Model file for the job. Use its own axes, mm. A direction names the side the tool comes from. Round coordinates to 2 decimals unless told otherwise and drop trailing zeros. Order: outer loops, then holes, each group sorted by start corner. A loop starts at its lowest first (then second) coordinate and runs counter-clockwise, first axis right, second up. Notation, with made-up numbers: (-2.5, -26) - (39.5, -26) arc R22 cw to (39.5, 5) - close; hole circle Ø6 at (51, -26). An arc over 180 degrees is marked (long way). Write item = value, one per line.
```python
from build123d import *

# Parameters (mm, degrees)
F0_W      = 19
F0_H      = 19
F1_DEPTH  = 9.5
F3_DEPTH  = 19.001
F5_DEPTH  = 3
F6_R      = 2
F8_DEPTH  = 12.501
F9_R      = 2
F11_DEPTH = 9.5
F12_R     = 2.99999
F13_R     = 2


# Not quite as in the source:
# - a fillet or chamfer is up to 0.001 mm smaller than in the source, because OpenCascade refuses the exact size


with BuildPart() as f1:
    # F0 (on Front) → F1 (new body, symmetric)
    with BuildSketch(Plane.XZ):
        with Locations((9.5, 9.5)):
            Rectangle(F0_W, F0_H)
    extrude(amount=F1_DEPTH, both=True)

    # F2 (on face) → F3 (cut, through all)
    with BuildSketch(Plane.XZ.offset(9.5)):
        with BuildLine():
            ThreePointArc((6, 19), (9.8076118446, 9.8076118446), (19, 6))
            Line((19, 6), (19, 19))
            Line((19, 19), (6, 19))
        make_face()
    extrude(amount=-F3_DEPTH, mode=Mode.SUBTRACT)

    # F4 (on Front) → F5 (join, symmetric)
    with BuildSketch(Plane.XZ):
        Polygon((0, 18), (0, 0), (18, 0), (18, 11.5), (24.5, 11.5), (24.5, 24.5), (11.5, 24.5), (11.5, 18), align=None)
    extrude(amount=F5_DEPTH, both=True)

    # F6
    f6_edges = [f1.edges().sort_by_distance(p)[0] for p in [
        (0, 0, 0),
    ]]
    fillet(f6_edges, radius=F6_R)

    # F7 (on face) → F8 (cut, through all)
    with BuildSketch(Plane.XZ.offset(3)):
        Polygon((17.5, 24.5), (24.5, 17.5), (24.5, 24.5), align=None)
    extrude(amount=-F8_DEPTH, mode=Mode.SUBTRACT)

    # F9
    f9_edges = [f1.edges().sort_by_distance(p)[0] for p in [
        (0, -9.5, 10.5),
        (0, 9.5, 10.5),
        (0, 0, 19),
        (3, 9.5, 19),
        (3, -9.5, 19),
        (19, 9.5, 3),
        (19, 0, 0),
        (19, -9.5, 3),
    ]]
    fillet(f9_edges, radius=F9_R)

    # F10 (on Front) → F11 (cut, symmetric)
    with BuildSketch(Plane.XZ):
        Polygon((0, 25), (0, 0), (25, 25), align=None)
    extrude(amount=F11_DEPTH, both=True, mode=Mode.SUBTRACT)

    # F12 (radius 3 in the source; OpenCascade refuses exactly that, so slightly less here)
    f12_edges = [f1.edges().sort_by_distance(p)[0] for p in [
        (22.75, -3, 19.25),
        (24.5, -3, 14.5),
        (24.5, 3, 14.5),
        (22.75, 3, 19.25),
    ]]
    fillet(f12_edges, radius=F12_R)

    # F13
    f13_edges = [f1.edges().sort_by_distance(p)[0] for p in [
        (23.579023, 2.162797, 17.118519),
    ]]
    fillet(f13_edges, radius=F13_R)


solid = f1.part
```
1) Cut at A-A (x = 6.5). Write the cut outline in (y, z).
Conclusion:
outline = (-9.5, 2) arc R2 ccw to (-7.5, 0) - (7.5, 0) arc R2 ccw to (9.5, 2) - (9.5, 6.5) - (-9.5, 6.5) - close
2) Cut at D-D (z = 7.5). Write the cut outline in (x, y), and give its area (3 significant figures).
Conclusion:
outline = (7.5, -9.5) - (12.94, -9.5) - (12.94, -3) - (18, -3) - (18, 3) - (12.94, 3) - (12.94, 9.5) - (7.5, 9.5) - close
area = 134 mm^2
3) Wall check: line 1 along Y through (x, z) = (19.75, 15.5); line 2 along Z through (x, y) = (11.5, -2.5); line 3 along Z through (x, y) = (6, -6). Give the ranges that are in metal, low to high.
Conclusion:
line_1 = -3 to 3
line_2 = 0 to 11.5
line_3 = 0 to 6
4) Cut at C-C (x = 15.75). Write the cut outline in (y, z), and give its area (3 significant figures).
Conclusion:
outline = (-9.5, 2) arc R2 ccw to (-7.5, 0) - (7.5, 0) arc R2 ccw to (9.5, 2) - (9.5, 6.41) - (3, 6.41) - (3, 15.75) - (-3, 15.75) - (-3, 6.41) - (-9.5, 6.41) - close
area = 176 mm^2
5) Mould opens along Z. For faces 6 (the face through (18, 0, 9)), 7 (the face through (9.4, -8.9, 0.57)), 8 (the face through (21.84, -2.145, 18.885)), 9 (the face through (11, 9.5, 5)) say: +Z half, -Z half, draft (parallel to the pull), parting line (faces both ways), or undercut.
Conclusion:
face_6 = undercut
face_7 = -Z half
face_8 = +Z half
face_9 = draft
6) Flat gauge pins, fed straight in: pin 1 Ø8 at (y, z) = (2.5, 3) entering from +X; pin 2 Ø12 at (x, z) = (16.5, 17.5) entering from +Y; pin 3 Ø5 at (x, y) = (22, 1.5) entering from -Z. Where does each tip first touch, or does it go through?
Conclusion:
pin_1 = 19
pin_2 = 3
pin_3 = 11.5
7) 3-axis set-ups, long thin cutter, end or side, ignore diameter. For faces 1 (the face through (19, 0, 4)), 2 (the face through (17, -3, 13)), 3 (the face through (21, 0, 11.5)), 4 (the face through (17, 3, 13)), 5 (the face through (9, 0, 0)): which of +Z, -Z, +X, -X, +Y, -Y reach the whole face in a straight line?
Conclusion:
face_1 = -Z, +X, +Y, -Y
face_2 = +Z, +X, -Y
face_3 = +X, +Y, -Y
face_4 = +Z, +X, +Y
face_5 = -Z, +X, -X, +Y, -Y
